```python
from build123d import *

# Parameters (mm, degrees)
F1_DEPTH = 3.175
F3_DEPTH = 25.4


# Not quite as in the source:
# - a feature of the source that left no trace in its solid (it failed there, or was rolled back) is left out


with BuildPart() as f1:
    # F0 (on Front) → F1 (new body)
    with BuildSketch(Plane.XZ):
        Polygon((83.7385465681, 60.7950414864), (65.4867140893, 43.1201200129), (42.6659945136, 31.9511005402), (48.4525043638, 20.1278488249), (53.8348904797, 9.1303205178), (53.9749918148, 8.1434892953), (55.6890408221, -3.9297509459), (57.4061805077, -16.0247609861), (82.5613006616, -12.4537432078), (107.5886724448, -16.8312881314), (111.9661336404, 8.1960982966), (123.863112913, 30.645911706), (101.4134680417, 42.5432090075), align=None)
        Polygon((62.8005820601, -8.8453070311), (59.98049806, 11.018507533), (51.1609480861, 29.0390003787), (69.1816050409, 37.8587515602), (83.5943604063, 51.8159429598), (97.5514190703, 37.4033246624), (115.278932926, 28.0085434102), (105.884368679, 10.2808320666), (102.427683451, -9.4821750964), (82.6646160624, -6.0254111952), align=None, mode=Mode.SUBTRACT)
        with BuildLine():
            Line((48.4525043638, 20.1278488249), (42.6659945136, 31.9511005402))
            ThreePointArc((42.6659945136, 31.9511005402), (8.9754555579, 27.0708614751), (-23.3620781244, 16.433518583))
            ThreePointArc((-23.3620781244, 16.433518583), (-83.2539454778, 3.5037557836), (-143.6249151078, 13.9708741582))
            add(Edge.make_bspline(
                [(-143.6249151078, 13.9708741582), (-139.3821490751, 9.1987873198), (-135.7140854359, 2.9639524936), (-137.4607610868, -0.5827256571), (-137.6279600012, -0.8521879559)],
                knots=[0, 0, 0, 0, 0.2240060147, 0.243416319, 0.243416319, 0.243416319, 0.243416319], degree=3))
            ThreePointArc((-137.6279600012, -0.8521879559), (-77.5676001001, -8.3586658465), (-18.6118863058, 5.3459995187))
            ThreePointArc((-18.6118863058, 5.3459995187), (14.224158407, 15.8953190594), (48.4525043638, 20.1278488249))
        make_face()
        with BuildLine():
            Line((53.8348904797, 9.1303205178), (48.4525043638, 20.1278488249))
            ThreePointArc((48.4525043638, 20.1278488249), (14.224158407, 15.8953190594), (-18.6118863058, 5.3459995187))
            ThreePointArc((-18.6118863058, 5.3459995187), (-77.5676001001, -8.3586658465), (-137.6279600012, -0.8521879559))
            add(Edge.make_bspline(
                [(-137.6279600012, -0.8521879559), (-138.9540636818, -2.9893725644), (-143.6991899879, -4.9863421871), (-144.9043234797, -9.4137473987), (-145.0020824108, -11.1490770117)],
                knots=[0.243416319, 0.243416319, 0.243416319, 0.243416319, 0.3973651411, 0.4804221604, 0.4804221604, 0.4804221604, 0.4804221604], degree=3))
            ThreePointArc((-145.0020824108, -11.1490770117), (-78.9349092151, -20.4976327315), (-13.8616894677, -5.7415173951))
            ThreePointArc((-13.8616894677, -5.7415173951), (19.3499940642, 4.6534346359), (53.9749918148, 8.1434892953))
            Line((53.9749918148, 8.1434892953), (53.8348904797, 9.1303205178))
        make_face()
        with BuildLine():
            Line((55.6890408221, -3.9297509459), (53.9749918148, 8.1434892953))
            ThreePointArc((53.9749918148, 8.1434892953), (19.3499940642, 4.6534346359), (-13.8616894677, -5.7415173951))
            ThreePointArc((-13.8616894677, -5.7415173951), (-78.9349092151, -20.4976327315), (-145.0020824108, -11.1490770117))
            add(Edge.make_bspline(
                [(-145.0020824108, -11.1490770117), (-145.148620527, -13.7502913411), (-144.2433778815, -18.4324653045), (-142.4737649258, -23.1788138286), (-141.761803512, -24.8017401992)],
                knots=[0.4804221604, 0.4804221604, 0.4804221604, 0.4804221604, 0.6049224901, 0.6738209053, 0.6738209053, 0.6738209053, 0.6738209053], degree=3))
            ThreePointArc((-141.761803512, -24.8017401992), (-74.7426386358, -32.3624002943), (-9.11149777, -16.8290365111))
            ThreePointArc((-9.11149777, -16.8290365111), (22.6146775302, -6.9930314551), (55.6890408221, -3.9297509459))
        make_face()
        with BuildLine():
            Line((57.4061805077, -16.0247609861), (55.6890408221, -3.9297509459))
            ThreePointArc((55.6890408221, -3.9297509459), (22.6146775302, -6.9930314551), (-9.11149777, -16.8290365111))
            ThreePointArc((-9.11149777, -16.8290365111), (-74.7426386358, -32.3624002943), (-141.761803512, -24.8017401992))
            add(Edge.make_bspline(
                [(-141.761803512, -24.8017401992), (-140.0858053256, -28.6222023777), (-135.8065528754, -35.5480454062), (-131.1858892441, -36.9351543486), (-130.136887087, -40.1733894927)],
                knots=[0.6738209053, 0.6738209053, 0.6738209053, 0.6738209053, 0.8360117443, 1, 1, 1, 1], degree=3))
            ThreePointArc((-130.136887087, -40.1733894927), (-66.2989601616, -43.7949576201), (-4.3613058839, -27.9165555465))
            ThreePointArc((-4.3613058839, -27.9165555465), (25.8820678715, -18.6444983253), (57.4061805077, -16.0247609861))
        make_face()
    extrude(amount=F1_DEPTH)

    # F2 (on Front) → F3 (cut)
    with BuildSketch(Plane.XZ):
        Polygon((56.6531529851, -10.7206639914), (53.8348904797, 9.1303205178), (45.7340942467, 25.6822240721), (44.3082079533, 24.9843699385), (52.2984898455, 8.6582741514), (55.0814150388, -10.9438050714), align=None)
    extrude(amount=F3_DEPTH, mode=Mode.SUBTRACT)


solid = f1.part
```
Check sheet for the modelled part. Datum: model origin and axes. Units: mm. A direction names the side the tool comes from. Round coordinates to 2 decimals unless told otherwise and drop trailing zeros. Loops run counter-clockwise (first coordinate to the right, second up) from the corner with the lowest first, then second, coordinate; pieces in that order, holes last. Notation, with made-up numbers: M 57,24.5 L 69,24.5 A10 ccw 69,41.5 Z; hole C -26,46 d3. An arc over 180 degrees is marked long. Answer as a JSON object with one key per item and string values.
1. Section check C-C (x = -77). Record the boundary of the cut face in (y, z) (3 decimals).
Reply:
{"outline": "M -3.175,-44.561 L 0,-44.561 L 0,3.754 L -3.175,3.754 Z"}
2. Access from +Z, -Z, +X, -X, +Y, -Y to the whole of each face (thin tool, end or side, straight path). Record for faces 1 (the flat face through (74.74, -1.57, 52.08)), 2 (the flat face through (94.9, -1.57, -14.61)), 3 (the flat face through (48.247, -1.565, 16.936)).
Reply:
{"face 1": "+Z, -X, +Y, -Y", "face 2": "-Z, +Y, -Y", "face 3": "+Y, -Y"}
3. Section check B-B (y = -2.2). State how many separate pieces and enclosed holes the cut face has, plus the area to 3 significant figures.
Reply:
{"separate pieces": "1", "enclosed holes": "2", "area": "10,900 mm²"}
4. Section check D-D (x = -106). Record the boundary of the cut face in (y, z) (3 decimals).
Reply:
{"outline": "M -3.175,-43.869 L 0,-43.869 L 0,4.655 L -3.175,4.655 Z"}
5. Gauge pin test, flat ends, axial feed: P1, Ø1, axis at x = -65, y = -1, coming from the +Z side; P2, Ø8, axis at x = 9.5, z = 32.5, coming from the -Y side; P3, Ø1.5, axis at x = 11, y = -1, coming from the +Z side; P4, Ø1.5, axis at x = -40, y = -1, coming from the -Z side. Record the tip position at first contact, or that the pin passes through.
Reply:
{"P1": "stops at z = 4.99", "P2": "passes through", "P3": "stops at z = 27.7", "P4": "stops at z = -39.69"}
6. Scan lines: line 1 (X direction, y = -2.55, z = 2); line 2 (X direction, y = -2.05, z = 0); line 3 (X direction, y = -1.8, z = 32). Record each from-to range of solid material in increasing order.
Reply:
{"line 1": "x = -136.98 to 53.24, 54.85 to 61.26, 104.44 to 110.88", "line 2": "x = -137.22 to 53.53, 55.13 to 61.54, 104.09 to 110.53", "line 3": "x = 42.77 to 57.21, 107.75 to 121.31"}
7. Mould release check, pull along X, two halves, no side actions. Record for faces 4 (the flat face through (54.236, -1.565, 37.614)), 5 (the flat face through (76.29, -1.57, 44.74)), 6 (the flat face through (112.8, -1.57, 36.51)), 7 (the cylindrical face through (25.45, -1.57, -18.73)): pulls with the +X half, pulls with the -X half, needs draft (parallel to the pull), parting line crosses it, or undercut.
Reply:
{"face 4": "pulls with the -X half", "face 5": "undercut", "face 6": "pulls with the +X half", "face 7": "undercut"}
8. Section check A-A (z = 47). Record the boundary of the cut face in (x, y) (3 decimals), plus the area to 3 significant figures.
Reply:
{"outline": "M 69.493,-3.175 L 78.621,-3.175 L 78.621,0 L 69.493,0 Z; M 88.258,-3.175 L 97.098,-3.175 L 97.098,0 L 88.258,0 Z", "area": "57.0 mm²"}
